Check sheet for the modelled part. Datum: model origin and axes. Units: mm. Give positions to 0.01 mm unless a question says otherwise; leave off trailing zeros. Write each loop counter-clockwise with the first axis right and the second up, starting at its lowest first coordinate (ties: lowest second). Pieces come first, ordered by that corner, then holes. Notation, with made-up numbers: M 58.25,-11 L 83.25,-11 A18 cw 83.25,19 Z; hole C 69.25,65.25 d8. An arc over 180 degrees is marked long. Write item = value, one per line. Start each with the question number.
1) Go/stop test with flat-tipped pins: pin 1 (2 mm diameter, centred on x = 15, z = 2.5, fed in from -Y); pin 2 (3 mm diameter, centred on y = -22, z = 0.5, fed in from -X); pin 3 (1 mm diameter, centred on y = -28.5, z = -0.5, fed in from +X); pin 4 (1.5 mm diameter, centred on y = -11, z = -0.5, fed in from +X). Record where each tip stops, or that it passes through.
2) Cross-section at B-B, the plane x = 9.5. Record the cut outline in (y, z).
3) Cross-section at A-A, the plane z = -1.95. Record the cut outline in (x, y).
4) Cross-section at C-C, the plane y = -2.5. Record the cut outline in (x, z).
5) Scan lines: line 1 along X through (y, z) = (-10.5, -0.6); line 2 along Y through (x, z) = (33.5, 0.5); line 3 along Y through (x, z) = (17.5, -2.2). Record each from-to range of solid material in increasing order. Write a range as [from, to].
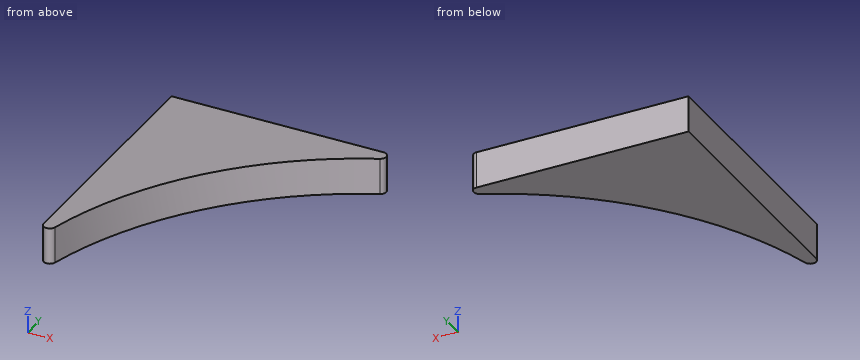
```python
from build123d import *

# Parameters (mm, degrees)
BOSS_EXTRUDE1_DEPTH     = 3
CUT_EXTRUDE1_DEPTH      = 73.173402303
CUT_EXTRUDE1_DEPTH_BACK = 73.173402303
FILLET1_R               = 1


with BuildPart() as part:
    # Sketch1 → Boss-Extrude1 (new, symmetric)
    with BuildSketch(Plane.XY):
        Polygon((0, 0), (0, -60), (40, 0), align=None)
    extrude(amount=BOSS_EXTRUDE1_DEPTH, both=True)

    # Sketch2 → Cut-Extrude1 (cut, two sides: drawn at the far end of the back side and taken through both)
    with BuildSketch(Plane.XY.offset(-CUT_EXTRUDE1_DEPTH_BACK)):
        with BuildLine():
            Line((40, 0), (0, -60))
            ThreePointArc((0, -60), (9.980712645, -23.320475097), (40, 0))
        make_face()
    extrude(amount=CUT_EXTRUDE1_DEPTH + CUT_EXTRUDE1_DEPTH_BACK, mode=Mode.SUBTRACT)

    # Fillet1
    fillet1_edges = [part.edges().sort_by_distance(p)[0] for p in [
        (0, -53.204973741, 0),
        (40, 0, 0),
    ]]
    fillet(fillet1_edges, radius=FILLET1_R)


solid = part.part
```
Reply:
q1.pin_1 = -17.97
q1.pin_2 = 0
q1.pin_3 = 7.16
q1.pin_4 = 21.81
q2.outline = M -24.05,-3 L 0,-3 L 0,3 L -24.05,3 Z
q3.outline = M 0,-40.75 A1 ccw 1.97,-41.01 A60 cw 35.23,-1.91 A1 ccw 34.82,0 L 0,0 Z
q4.outline = M 0,-3 L 33.96,-3 L 33.96,3 L 0,3 Z
q5.line_1 = [0, 21.5]
q5.line_2 = [-2.72, 0]
q5.line_3 = [-14.15, 0]
